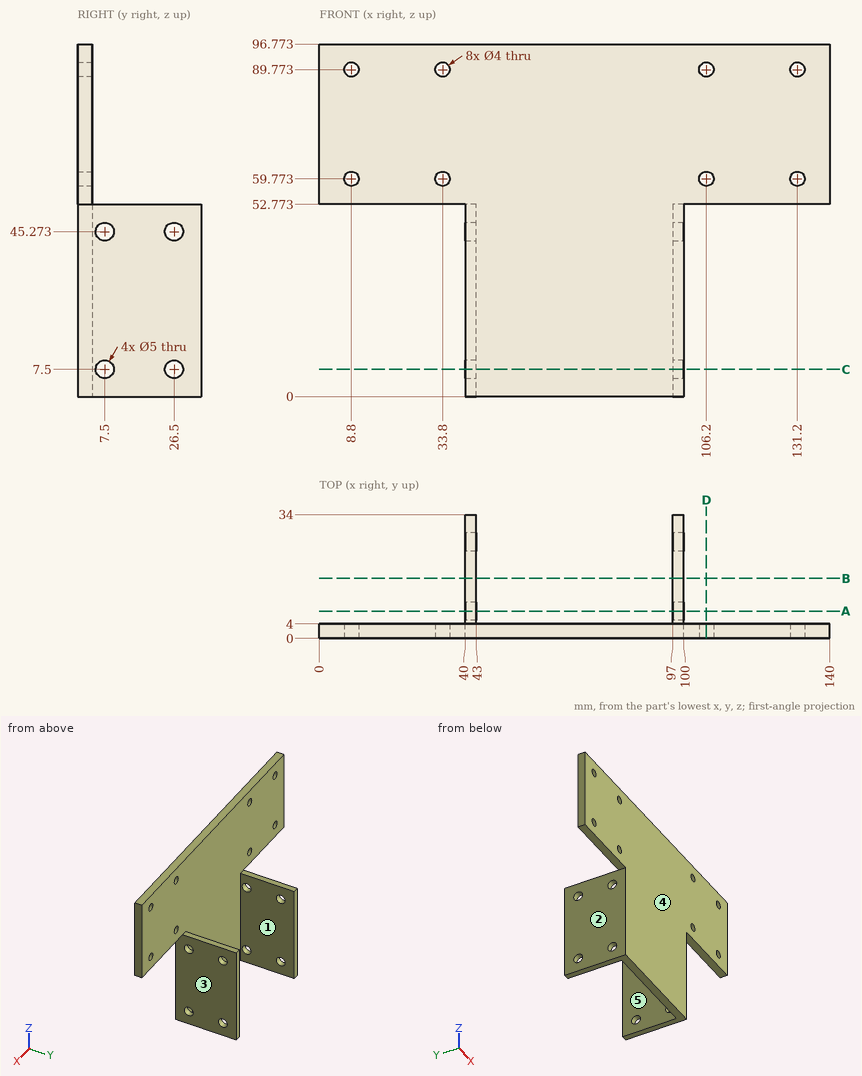
Geometry check sheet. Reference: drawing and pictorial views, mm from the part's lowest x, y, z. A direction names the side the tool comes from. Round coordinates to 2 decimals unless told otherwise and drop trailing zeros. Loops run counter-clockwise (first coordinate to the right, second up) from the corner with the lowest first, then second, coordinate; pieces in that order, holes last. Notation, with made-up numbers: (39, -30) -> (76, -30) arc R12 cw to (76, -8) -> close; hole circle Ø3 at (2, 13). An arc over 180 degrees is marked (long way). Answer as a JSON object with one key per item and string values. Group by question number.
Item 1: Cross-section at A-A, the plane y = 7.5. Record the cut outline in (x, z).
Item 2: Release check for a two-part mould opening along X. For the marked faces 3, 4 and 5 record: pulls with the +X half, pulls with the -X half, needs draft (parallel to the pull), parting line crosses it, or undercut.
Item 3: Cross-section at D-D, the plane x = 106.2. Record the cut outline in (y, z), plus the area to 3 significant figures.
Item 4: Set-up check for the marked faces 1 and 2: record each of +Z, -Z, +X, -X, +Y, -Y from which the full face is reachable in a straight line by a thin tool's end or side.
Item 5: Thickness scan on line 1 along Z through (x, y) = (40.9, 7.5); line 2 along X through (y, z) = (29, 27); line 3 along Y through (x, z) = (99, 7). Record the ranges inside material, lowest first.
Item 6: Cross-section at B-B, the plane y = 16.5. Record the cut outline in (x, z).
Item 7: Depth check by flat-ended pin: pin 1 Ø3.5 at (x, z) = (131.2, 59.77) entering from +Y; pin 2 Ø6 at (y, z) = (7.5, 45.27) entering from +X; pin 3 Ø6.5 at (x, z) = (33.8, 59.77) entering from -Y; pin 4 Ø15 at (y, z) = (23.5, 30) entering from -X. Enter the tip coordinate at first touch or a pass-through.
Item 8: Cross-section at C-C, the plane z = 7.5. Record the cut outline in (x, y).
Determined:
{
 "1": {"outline": "(40, 0) -> (43, 0) -> (43, 5) -> (40, 5) -> close; (40, 10) -> (43, 10) -> (43, 42.77) -> (40, 42.77) -> close; (40, 47.77) -> (43, 47.77) -> (43, 52.77) -> (40, 52.77) -> close; (97, 0) -> (100, 0) -> (100, 5) -> (97, 5) -> close; (97, 10) -> (100, 10) -> (100, 42.77) -> (97, 42.77) -> close; (97, 47.77) -> (100, 47.77) -> (100, 52.77) -> (97, 52.77) -> close"},
 "2": {"face 3": "pulls with the +X half", "face 4": "needs draft", "face 5": "undercut"},
 "3": {"outline": "(0, 52.77) -> (4, 52.77) -> (4, 57.77) -> (0, 57.77) -> close; (0, 61.77) -> (4, 61.77) -> (4, 87.77) -> (0, 87.77) -> close; (0, 91.77) -> (4, 91.77) -> (4, 96.77) -> (0, 96.77) -> close", "area": "144 mm²"},
 "4": {"face 1": "+Z, -Z, +Y", "face 2": "-Z, -X, +Y, -Y"},
 "5": {"line 1": "z = 0 to 5, 10 to 42.77, 47.77 to 52.77", "line 2": "x = 40 to 43, 97 to 100", "line 3": "y = 0 to 5.05, 9.95 to 24.05, 28.95 to 34"},
 "6": {"outline": "(40, 0) -> (43, 0) -> (43, 52.77) -> (40, 52.77) -> close; (97, 0) -> (100, 0) -> (100, 52.77) -> (97, 52.77) -> close"},
 "7": {"pin 1": "passes through", "pin 2": "stops at x = 100", "pin 3": "stops at y = 0", "pin 4": "stops at x = 40"},
 "8": {"outline": "(40, 0) -> (100, 0) -> (100, 5) -> (97, 5) -> (97, 4) -> (43, 4) -> (43, 5) -> (40, 5) -> close; (40, 10) -> (43, 10) -> (43, 24) -> (40, 24) -> close; (40, 29) -> (43, 29) -> (43, 34) -> (40, 34) -> close; (97, 10) -> (100, 10) -> (100, 24) -> (97, 24) -> close; (97, 29) -> (100, 29) -> (100, 34) -> (97, 34) -> close"}
}
